The model under review builds one solid part; all positions refer to its coordinate system, in mm. A direction names the side the tool comes from. Coordinates: 2 decimals unless noted, no trailing zeros. Loops run counter-clockwise (first coordinate to the right, second up) from the corner with the lowest first, then second, coordinate; pieces in that order, holes last. Notation, with made-up numbers: (26.5, 82.25) -> (54.5, 82.25) arc R18 cw to (54.5, 115.25) -> close; hole circle Ø7 at (-1, -11). An arc over 180 degrees is marked (long way). One line per question, with ' | ' between items. Start each with the question number.
from build123d import *

# Parameters (mm, degrees)
EXTRUDE_1_DEPTH     = 255
SKETCH_2_R          = 5
CUT_EXTRUDE_1_DEPTH = 44


with BuildPart() as part:
    # Эскиз1 → Вытянуть-Тонкостенный1 (new body)
    with BuildSketch(Plane(origin=(0, 0, 0), x_dir=(0, 0, -1), z_dir=(1, 0, 0))):
        Polygon((0, 43), (0, 0), (43, 0), (43, 4), (4, 4), (4, 43), align=None)
    extrude(amount=EXTRUDE_1_DEPTH)

    # Эскиз2 → Вырез-Вытянуть1 (cut, through all)
    with BuildSketch(Plane.XZ):
        with Locations((80, -23)):
            Circle(SKETCH_2_R)
        with Locations((180, -23)):
            Circle(SKETCH_2_R)
    extrude(amount=-CUT_EXTRUDE_1_DEPTH, mode=Mode.SUBTRACT)


solid = part.part
1) Machinability: for faces 1 (the face through (126, 2, -43)), 2 (the face through (126, 4, -24)), which of the approach directions +Z, -Z, +X, -X, +Y, -Y give a long, thin tool a straight path to every point of the face, cutting with its end or side? Answer none if there is none.
2) Mouldability with a two-part tool opening along Z and no side actions: class faces 3 (the face through (176, 2, -26)), 4 (the face through (126, 22, 0)), 5 (the face through (255, 14, -2)) as +Z half, -Z half, draft (parallel to the pull), parting line (faces both ways), or undercut.
3) Consider section B-B, the plane z = -23. Write out the cut boundary in (x, y), plus the area to 3 significant figures.
4) Consider section D-D, the plane z = -33. Write out the cut boundary in (x, y), plus the area to 3 significant figures.
5) Wall thickness on L1, parallel to Z at x = 180, y = 1.35; L2, parallel to Z at x = 115.5, y = 18.5; L3, parallel to X at y = 3, z = -21.5: over which ranges is each line inside the solid? List them lowest first.
6) Consider section A-A, the plane x = 180. Write out the cut boundary in (y, z), plus the area to 3 significant figures.
7) Insertion check: pin 1 Ø13 at (x, z) = (180, -23) entering from +Y; pin 2 Ø3 at (x, y) = (180, 25) entering from -Z; pin 3 Ø12 at (y, z) = (15.5, -21) entering from +X. Each pin has a flat end and moves straight along its axis. Give the tip position at first contact, or say it passes through.
8) Consider section C-C, the plane y = 30. Write out the cut boundary in (x, z).
Filled sheet:
1) face 1: -Z, +X, -X, +Y, -Y | face 2: -Z, +X, -X, +Y
2) face 3: undercut | face 4: +Z half | face 5: draft
3) outline: (0, 0) -> (75, 0) -> (75, 4) -> (0, 4) -> close; (85, 0) -> (175, 0) -> (175, 4) -> (85, 4) -> close; (185, 0) -> (255, 0) -> (255, 4) -> (185, 4) -> close | area: 940 mm^2
4) outline: (0, 0) -> (255, 0) -> (255, 4) -> (0, 4) -> close | area: 1,020 mm^2
5) L1: -43 to -28, -18 to 0 | L2: -4 to 0 | L3: 0 to 75.23, 84.77 to 175.23, 184.77 to 255
6) outline: (0, -43) -> (4, -43) -> (4, -28) -> (0, -28) -> close; (0, -18) -> (4, -18) -> (4, -4) -> (43, -4) -> (43, 0) -> (0, 0) -> close | area: 288 mm^2
7) pin 1: y = 4 | pin 2: z = -4 | pin 3: through
8) outline: (0, -4) -> (255, -4) -> (255, 0) -> (0, 0) -> close
